```python
from build123d import *

# Parameters (mm, degrees)
SKETCH1_W               = 16
SKETCH1_H               = 38.42
BOSS_EXTRUDE1_DEPTH     = 2
SKETCH2_W               = 9.5
SKETCH2_H               = 31.92
SKETCH2_W_2             = 6.5
SKETCH2_H_2             = 28.92
EXTRUDE_THIN1_DEPTH     = 1
SKETCH3_R               = 1
CUT_EXTRUDE1_DEPTH      = 4
MIRROR2_COPY_1_SKETCH_R = 1
MIRROR2_COPY_1_DEPTH    = 4
SKETCH5_R               = 0.75
CUT_EXTRUDE2_DEPTH      = 2
CUT_EXTRUDE2_DEPTH_BACK = 3
SKETCH6_R               = 1.25
CUT_EXTRUDE6_DEPTH      = 0.5
SKETCH7_R               = 1.5
BOSS_EXTRUDE2_DEPTH     = 1
SKETCH9_R               = 0.25
CUT_EXTRUDE7_DEPTH      = 2


with BuildPart() as part:
    # Sketch1 → Boss-Extrude1 (new body)
    with BuildSketch(Plane(origin=(0, 0, 0), x_dir=(1, 0, 0), z_dir=(0, 1, 0))):
        Rectangle(SKETCH1_W, SKETCH1_H)
    extrude(amount=BOSS_EXTRUDE1_DEPTH)

    # Sketch2 → Extrude-Thin1 (add)
    with BuildSketch(Plane(origin=(0, 2, 0), x_dir=(1, 0, 0), z_dir=(0, 1, 0))):
        Rectangle(SKETCH2_W, SKETCH2_H)
        Rectangle(SKETCH2_W_2, SKETCH2_H_2, mode=Mode.SUBTRACT)
    extrude(amount=EXTRUDE_THIN1_DEPTH)

    # Sketch3 → Cut-Extrude1 (cut, through all)
    with BuildSketch(Plane.XZ):
        with Locations((6, 17.21)):
            Circle(SKETCH3_R)
    cut_extrude1 = extrude(amount=-CUT_EXTRUDE1_DEPTH, mode=Mode.SUBTRACT)

    # Mirror1: Cut-Extrude1 across plane
    add(cut_extrude1.mirror(Plane(origin=(0, 0, 0), x_dir=(1, 0, 0), z_dir=(0, 0, -1))), mode=Mode.SUBTRACT)

    # Mirror2: Cut-Extrude1 across plane
    add(cut_extrude1.mirror(Plane.ZY), mode=Mode.SUBTRACT)

    # Mirror2 copy 1 sketch → Mirror2 copy 1 (cut, through all)
    with BuildSketch(Plane(origin=(0, 0, 0), x_dir=(-1, 0, 0), z_dir=(0, -1, 0))):
        with Locations((6, 17.21)):
            Circle(MIRROR2_COPY_1_SKETCH_R)
    extrude(amount=-MIRROR2_COPY_1_DEPTH, mode=Mode.SUBTRACT)

    # Sketch5 → Cut-Extrude2 (cut, two sides)
    with BuildSketch(Plane(origin=(0, 2, 0), x_dir=(1, 0, 0), z_dir=(0, 1, 0))) as cut_extrude2_sk:
        Circle(SKETCH5_R)
    extrude(amount=CUT_EXTRUDE2_DEPTH, mode=Mode.SUBTRACT)
    extrude(cut_extrude2_sk.sketch, amount=-CUT_EXTRUDE2_DEPTH_BACK, mode=Mode.SUBTRACT)

    # Sketch6 → Cut-Extrude6 (cut)
    with BuildSketch(Plane(origin=(0, 2, 0), x_dir=(1, 0, 0), z_dir=(0, 1, 0))):
        Circle(SKETCH6_R)
    extrude(amount=-CUT_EXTRUDE6_DEPTH, mode=Mode.SUBTRACT)

    # Sketch7 → Boss-Extrude2 (add)
    with BuildSketch(Plane.XZ):
        Circle(SKETCH7_R)
    extrude(amount=BOSS_EXTRUDE2_DEPTH)

    # Sketch9 → Cut-Extrude7 (cut)
    with BuildSketch(Plane.XZ.offset(1)):
        Circle(SKETCH9_R)
    extrude(amount=-CUT_EXTRUDE7_DEPTH, mode=Mode.SUBTRACT)


solid = part.part
```
CAD build for the part. Positions are in the model's coordinates, mm. A direction names the side the tool comes from. Round coordinates to 2 decimals unless told otherwise and drop trailing zeros. Order: outer loops, then holes, each group sorted by start corner. A loop starts at its lowest first (then second) coordinate and runs counter-clockwise, first axis right, second up.
Q1. Slice it at B-B (x = -6). Write the cut outline in (y, z), and give its area (3 significant figures).
Q2. Slice it at A-A (z = 17.21). Write the cut outline in (x, y).
Q3. Slice it at D-D (y = 2.55). Write the cut outline in (x, z).
Q4. Two-plate mould, pull along Z, no slides. Class faces 6 (the flat face through (4.75, 2.5, 0.2)), 7 (the cylindrical face through (-1.5, -0.49, 0.07)), 8 (the cylindrical face through (-5.783, 0.986, 16.234)): pulls with the +Z half, pulls with the -Z half, needs draft (parallel to the pull), parting line crosses it, or undercut.
Q5. Which spindle directions (+Z, -Z, +X, -X, +Y, -Y) get a long thin tool onto all of the face, cutting with end or side? Do faces 1 (the flat face through (0, -1, 0.4)), 2 (the flat face through (-4.75, 2.5, 0.2)), 3 (the flat face through (-0.1, 2.5, -15.96)), 4 (the flat face through (-0.1, 2.5, 15.96)), 5 (the cylindrical face through (-0.27, 1.75, 1.22)). Say none if no direction does.
Q6. Drop flat-ended pins along their axis: pin 1 (0.8 mm diameter, centred on x = 0.5, y = 2.5, fed in from +Z); pin 2 (1.5 mm diameter, centred on x = 4, z = -12.5, fed in from -Y); pin 3 (0.8 mm diameter, centred on y = 2.5, z = 1.5, fed in from +X). Give the stop position or say it passes through.
Q7. Slice it at C-C (y = 1). Write the cut outline in (x, z).
Q8. Wall check: L1, parallel to Z at x = -6, y = 1.55; L2, parallel to Z at x = 0, y = 0.7; L3, parallel to X at y = 2.1, z = -12. Give the ranges that are in metal, low to high.
Results below:
1. outline: (0, -19.21) - (2, -19.21) - (2, -18.21) - (0, -18.21) - close; (0, -16.21) - (2, -16.21) - (2, 16.21) - (0, 16.21) - close; (0, 18.21) - (2, 18.21) - (2, 19.21) - (0, 19.21) - close
1. area: 68.8 mm2
2. outline: (-8, 0) - (-7, 0) - (-7, 2) - (-8, 2) - close; (-5, 0) - (5, 0) - (5, 2) - (-5, 2) - close; (7, 0) - (8, 0) - (8, 2) - (7, 2) - close
3. outline: (-4.75, -15.96) - (4.75, -15.96) - (4.75, 15.96) - (-4.75, 15.96) - close; hole (-3.25, -14.46) - (3.25, -14.46) - (3.25, 14.46) - (-3.25, 14.46) - close
4. face 6: needs draft
4. face 7: parting line crosses it
4. face 8: undercut
5. face 1: +Z, -Z, +X, -X, -Y
5. face 2: +Z, -Z, -X, +Y
5. face 3: -Z, +X, -X, +Y
5. face 4: +Z, +X, -X, +Y
5. face 5: +Y
6. pin 1: stops at z = 15.96
6. pin 2: stops at y = 0
6. pin 3: stops at x = 4.75
7. outline: (-8, -19.21) - (8, -19.21) - (8, 19.21) - (-8, 19.21) - close; hole circle Ø2 at (-6, -17.21); hole circle Ø2 at (-6, 17.21); hole circle Ø1.5 at (0, 0); hole circle Ø2 at (6, -17.21); hole circle Ø2 at (6, 17.21)
8. L1: z = -19.21 to -18.21, -16.21 to 16.21, 18.21 to 19.21
8. L2: z = -19.21 to -0.75, 0.75 to 19.21
8. L3: x = -4.75 to -3.25, 3.25 to 4.75
